```python
from build123d import *


with BuildPart() as part:
    # Sketch1 → Revolve-Thin1 (revolve)
    with BuildSketch(Plane.XY):
        with BuildLine():
            Line((2.159, 17.018), (2.159, 13.657028027))
            ThreePointArc((2.159, 13.657028027), (2.110446888, 13.309224203), (1.9685, 12.988014013))
            ThreePointArc((1.9685, 12.988014013), (1.826553112, 12.666803824), (1.778, 12.319))
            Line((1.778, 12.319), (1.778, 4.699))
            ThreePointArc((1.778, 4.699), (1.826553112, 4.351196176), (1.9685, 4.029985987))
            ThreePointArc((1.9685, 4.029985987), (2.110446888, 3.708775797), (2.159, 3.360971973))
            Line((2.159, 3.360971973), (2.159, 0))
            Line((2.159, 0), (1.397, 0))
            Line((1.397, 0), (1.397, 3.360971973))
            ThreePointArc((1.397, 3.360971973), (1.377578755, 3.500093503), (1.3208, 3.628577579))
            ThreePointArc((1.3208, 3.628577579), (1.093684979, 4.142513882), (1.016, 4.699))
            Line((1.016, 4.699), (1.016, 12.319))
            ThreePointArc((1.016, 12.319), (1.093684979, 12.875486118), (1.3208, 13.389422421))
            ThreePointArc((1.3208, 13.389422421), (1.377578755, 13.517906497), (1.397, 13.657028027))
            Line((1.397, 13.657028027), (1.397, 17.018))
            Line((1.397, 17.018), (2.159, 17.018))
        make_face()
    revolve(axis=Axis((0, 17.018, 0), (0, -1, 0)))


solid = part.part
```
Design review of the part built by this model. Coordinates are the model's own, in mm. A direction names the side the tool comes from. Round coordinates to 2 decimals unless told otherwise and drop trailing zeros. Order: outer loops, then holes, each group sorted by start corner. A loop starts at its lowest first (then second) coordinate and runs counter-clockwise, first axis right, second up. Notation, with made-up numbers: (-15, 45.5) - (-4, 45.5) arc R28 ccw to (-4, 66.5) - close; hole circle Ø4 at (21.5, 68). An arc over 180 degrees is marked (long way). Return JSON: item names as keys, results as strings.
Q1. Wall thickness on L1, parallel to X at y = 14, z = -0.05; L2, parallel to Z at x = -0.8, y = 3: over which ranges is each line inside the solid? List them lowest first. Write a range as [from, to].
Computed values:
{"L1": "x = [-2.16, -1.4], [1.4, 2.16]", "L2": "z = [-2.01, -1.15], [1.15, 2.01]"}
Q2. The part is to be moulded in two halves that separate along Y. For faces 1 (the cylindrical face through (-0.385, 8.456, -1.736)), 2 (the cylindrical face through (-1.11, 15.36, -0.85)), say which applies: pulls with the +Y half, pulls with the -Y half, needs draft (parallel to the pull), parting line crosses it, or undercut.
Computed values:
{"face 1": "undercut", "face 2": "needs draft"}
Q3. For pin 1 Ø2.5 at (x, z) = (0, 0) entering from -Y; pin 2 Ø1 at (x, y) = (-0.5, 7) entering from -Z; pin 3 Ø2 at (x, y) = (-0.5, 7) entering from +Z, all flat-tipped, find the tip position at first contact; note any pin that passes through.
Computed values:
{"pin 1": "stops at y = 3.75", "pin 2": "stops at z = -1.78", "pin 3": "stops at z = 1.78"}
Q4. Consider section B-B on y = 15.75. Write out the cut boundary in (x, z), plus the area to 3 significant figures.
Computed values:
{"outline": "circle Ø4.32 at (0, 0); hole circle Ø2.79 at (0, 0)", "area": "8.51 mm2"}
Q5. Consider section A-A on y = 10. Write out the cut boundary in (x, z).
Computed values:
{"outline": "circle Ø3.56 at (0, 0); hole circle Ø2.03 at (0, 0)"}
Q6. Machinability: for faces 3 (the cylindrical face through (-0.28, 15.31, 2.14)), 4 (the cylindrical face through (-1.11, 1.7, -0.85)), which of the approach directions +Z, -Z, +X, -X, +Y, -Y give a long, thin tool a straight path to every point of the face, cutting with its end or side? Answer none if there is none.
Computed values:
{"face 3": "+Y, -Y", "face 4": "-Y"}
